The figure shows three views and two pictorial views of one solid part (mm, origin at its lowest corner). Answer the questions. A direction names the side the tool comes from. Coordinates: 2 decimals unless noted, no trailing zeros. Order: outer loops, then holes, each group sorted by start corner. A loop starts at its lowest first (then second) coordinate and runs counter-clockwise, first axis right, second up. Notation, with made-up numbers: (22, -5) -> (58, -5) arc R25 cw to (58, 31) -> close; hole circle Ø4 at (3, -34). An arc over 180 degrees is marked (long way). Write item = value, one per line.
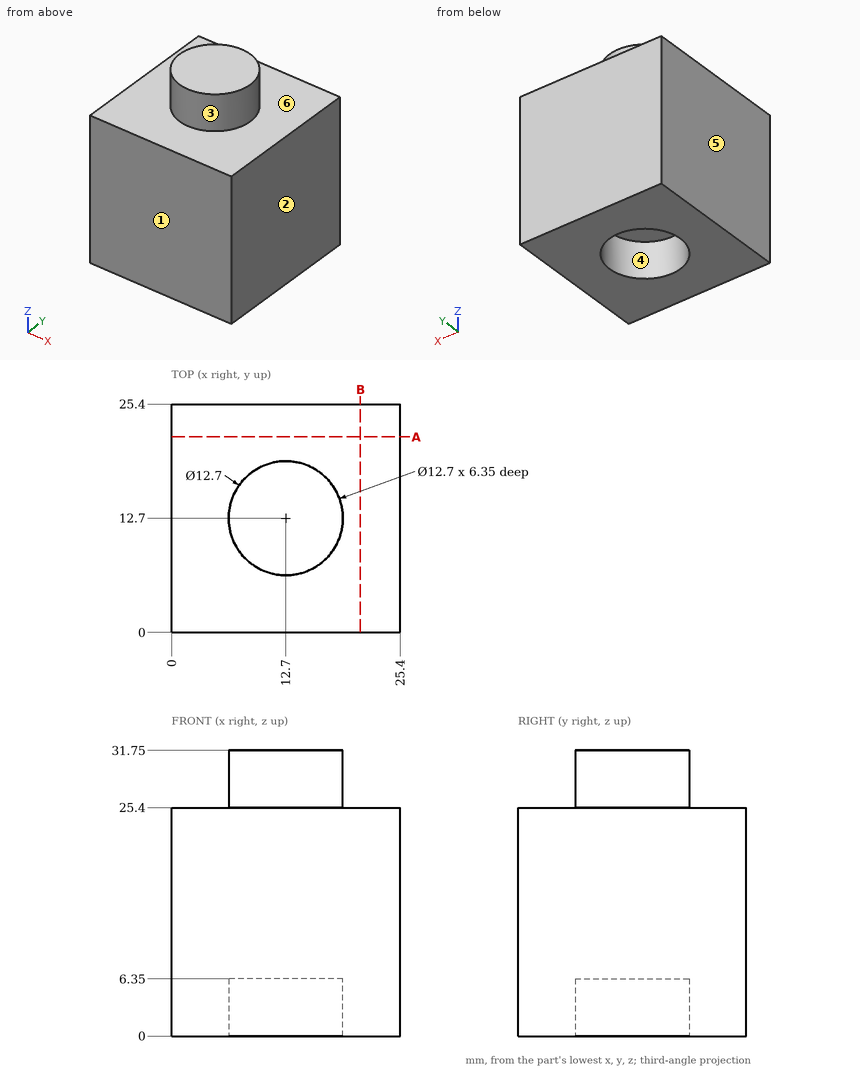
Q1. Find the intervals of material crossed by line 1 along Y through (x, z) = (12.7, 3.25); line 2 along Z through (x, y) = (18.5, 10.5), in increasing order.
The answers:
line_1 = 0 to 6.35, 19.05 to 25.4
line_2 = 6.35 to 31.75
Q2. Section A-A, the plane y = 21.75 is taken. Give the vertices of the cut face in (x, z).
The answers:
outline = (0, 0) -> (25.4, 0) -> (25.4, 25.4) -> (0, 25.4) -> close
Q3. This flat-tipped pin is pushed along its axis until it touches: pin 1 Ø3 at (y, z) = (10, 27) entering from -X. Where does it stop, or does it pass through?
The answers:
pin_1 = 6.46
Q4. A tool of negligible diameter and unlimited length cuts with its end or side. For the marked faces 5 and 6, from which of +Z, -Z, +X, -X, +Y, -Y can it reach the whole face along a straight path? Write none if from no direction.
The answers:
face_5 = +Z, -Z, -X, +Y, -Y
face_6 = +Z
Q5. The mould has two halves that part along Y. Classify the marked faces 1, 2, 3 and 4: released by +Y, released by -Y, zero draft, split by the parting line, or undercut.
The answers:
face_1 = released by -Y
face_2 = zero draft
face_3 = split by the parting line
face_4 = undercut
